from build123d import *

# Parameters (mm, degrees)
SKETCH1_R           = 15
BOSS_EXTRUDE1_DEPTH = 80
SKETCH2_R           = 10
BOSS_EXTRUDE2_DEPTH = 5
SKETCH3_R           = 2.5
BOSS_EXTRUDE3_DEPTH = 30
FILLET1_R           = 2
FILLET2_R           = 2
FILLET3_R           = 2
SKETCH4_R           = 7.5
BOSS_EXTRUDE5_DEPTH = 5
SKETCH5_R           = 2.5
BOSS_EXTRUDE6_DEPTH = 10
FILLET4_R           = 2


with BuildPart() as part:
    # Sketch1 → Boss-Extrude1 (new body)
    with BuildSketch(Plane(origin=(0, 0, 0), x_dir=(0, 0, -1), z_dir=(1, 0, 0))):
        Circle(SKETCH1_R)
    extrude(amount=BOSS_EXTRUDE1_DEPTH)

    # Sketch2 → Boss-Extrude2 (add)
    with BuildSketch(Plane(origin=(80, 0, 0), x_dir=(0, 0, -1), z_dir=(1, 0, 0))):
        Circle(SKETCH2_R)
    extrude(amount=BOSS_EXTRUDE2_DEPTH)

    # Sketch3 → Boss-Extrude3 (add)
    with BuildSketch(Plane(origin=(85, 0, 0), x_dir=(0, 0, -1), z_dir=(1, 0, 0))):
        Circle(SKETCH3_R)
    extrude(amount=BOSS_EXTRUDE3_DEPTH)

    # Fillet1
    fillet1_edges = [part.edges().sort_by_distance(p)[0] for p in [
        (80, 0, 15),
    ]]
    fillet(fillet1_edges, radius=FILLET1_R)

    # Fillet2
    fillet2_edges = [part.edges().sort_by_distance(p)[0] for p in [
        (85, 0, 10),
    ]]
    fillet(fillet2_edges, radius=FILLET2_R)

    # Fillet3
    fillet3_edges = [part.edges().sort_by_distance(p)[0] for p in [
        (0, 0, 15),
    ]]
    fillet(fillet3_edges, radius=FILLET3_R)

    # Sketch4 → Boss-Extrude5 (add)
    with BuildSketch(Plane.ZY):
        Circle(SKETCH4_R)
    extrude(amount=BOSS_EXTRUDE5_DEPTH)

    # Sketch5 → Boss-Extrude6 (add)
    with BuildSketch(Plane.ZY.offset(5)):
        Circle(SKETCH5_R)
    extrude(amount=BOSS_EXTRUDE6_DEPTH)

    # Fillet4
    fillet4_edges = [part.edges().sort_by_distance(p)[0] for p in [
        (115, 0, 2.5),
        (-15, 0, -2.5),
    ]]
    fillet(fillet4_edges, radius=FILLET4_R)


solid = part.part
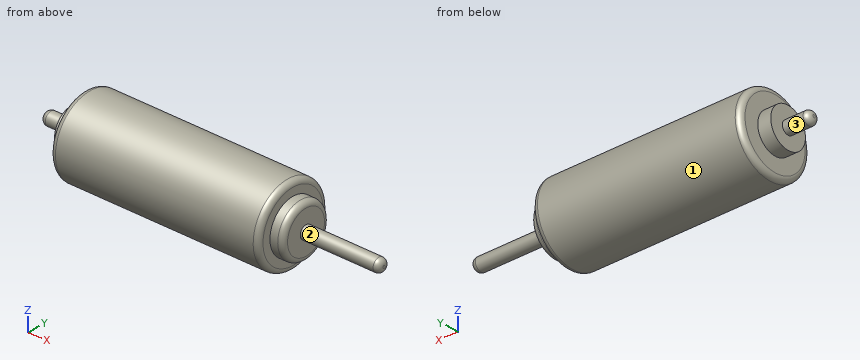
Geometry check sheet. Reference: the model listing, model coordinates, mm. Face numbers are marked on the shaded views. A direction names the side the tool comes from. Give positions to 0.01 mm unless a question says otherwise; leave off trailing zeros. Loops run counter-clockwise (first coordinate to the right, second up) from the corner with the lowest first, then second, coordinate; pieces in that order, holes last. Notation, with made-up numbers: M 26.25,4 L 72.25,4 A21 ccw 72.25,20 Z; hole C -30,54 d1. An arc over 180 degrees is marked long. Write each question's results on one line, items separated by ' | '.
1) Gauge pin test, flat ends, axial feed: pin 1 (4 mm diameter, centred on y = -9, z = -8, fed in from -X); pin 2 (1.5 mm diameter, centred on y = -3.5, z = -10.5, fed in from +X); pin 3 (10 mm diameter, centred on x = 93, z = -9.5, fed in from -Y); pin 4 (4 mm diameter, centred on y = -4, z = 2.5, fed in from +X). Record the tip position at first contact, or that the pin passes through.
Answers follow:
pin 1: x = 0 | pin 2: x = 80 | pin 3: through | pin 4: x = 85
2) Thickness scan on line 1 (X direction, y = -4.75, z = 9); line 2 (X direction, y = -2.25, z = -6); line 3 (Y direction, x = 3, z = -13). Record the ranges inside material, lowest first.
Answers follow:
line 1: 0 to 80 | line 2: -5 to 85 | line 3: -7.48 to 7.48
3) Section check B-B, the plane x = 88. Record the boundary of the cut face in (y, z).
Answers follow:
outline: C 0,0 d5
4) Section check A-A, the plane x = 64. Record the boundary of the cut face in (y, z).
Answers follow:
outline: C 0,0 d30
5) Tool access check on the marked faces 1, 2 and 3. Record the directions out of +Z, -Z, +X, -X, +Y, -Y that give a thin tool (end or side, any length) a straight path to the whole face; none if there is none.
Answers follow:
face 1: +X, -X | face 2: +X | face 3: -X
